For this review, take the finished solid that the model builds, in its own axes (mm). A direction names the side the tool comes from. Coordinates: 2 decimals unless noted, no trailing zeros. Loops run counter-clockwise (first coordinate to the right, second up) from the corner with the lowest first, then second, coordinate; pieces in that order, holes last. Notation, with made-up numbers: (8.25, 48) - (48.25, 48) arc R26 cw to (48.25, 80) - close; hole circle Ø7 at (-30, 49). An arc over 180 degrees is marked (long way). Use one line per item in the form item = value. Start each with the question number.
1. Machinability: for faces 4 (the face through (2.75, 10.74, -2.38)), 5 (the face through (2.5, -11, -2)), which of the approach directions +Z, -Z, +X, -X, +Y, -Y give a long, thin tool a straight path to every point of the face, cutting with its end or side? Answer none if there is none.
2. For pin 1 Ø6 at (y, z) = (-18.5, 0) entering from +X; pin 2 Ø1 at (x, z) = (3.5, -2) entering from -Y; pin 3 Ø4 at (y, z) = (-10, -3.5) entering from -X, all flat-tipped, find the tip position at first contact; note any pin that passes through.
3. To check wall thickness, follow probe 1 along Y at (x, z) = (1.8, 0); probe 2 along Z at (x, y) = (4.45, -1); probe 3 along Z at (x, y) = (2.9, 19.5). State the ranges of each line that lie inside material, in increasing order.
4. Draft analysis for pull direction Z (two halves, no side actions). For faces 1 (the face through (1.268, 12.864, 6.691)), 2 (the face through (2.218, -22.804, -2.994)), 3 (the face through (5, 10, -10)), state which applies: +Z half, -Z half, draft (parallel to the pull), parting line (faces both ways), or undercut.
5. Add section A-A on y = 0. Give the boundary of the cut face in (x, z).
6. Add section C-C on x = 1.7. Give the boundary of the cut face in (y, z), and give its area (3 significant figures).
```python
from build123d import *

# Parameters (mm, degrees)
SKETCH_2_R               = 2.25
CUT_EXTRUDE_1_DEPTH      = 33.908965344
PATTERN_CIRCULAR_1_COUNT = 4
CHAMFER_1_SIZE           = 0.5


with BuildPart() as part:
    # Эскиз1 → Повернуть1 (revolve)
    with BuildSketch(Plane.XY, mode=Mode.PRIVATE) as revolve_1_sk:
        Polygon((0, 23), (0, 14.5), (2.5, 14.5), (2.5, 11), (3, 11), (5, 13), (5, 23), align=None)
    revolve(revolve_1_sk.sketch.rotate(Axis((0, 0, 0), (1, 0, 0)), 90), axis=Axis((0, 0, 0), (1, 0, 0)))

    # Эскиз2 → Вырез-Вытянуть1 (cut, through all)
    with BuildSketch(Plane(origin=(5, 0, 0), x_dir=(0, 0, -1), z_dir=(1, 0, 0))):
        with Locations((0, 18.5)):
            Circle(SKETCH_2_R)
    cut_extrude_1 = extrude(amount=-CUT_EXTRUDE_1_DEPTH, mode=Mode.SUBTRACT)

    # Круговой массив1: Вырез-Вытянуть1 ×4 about axis
    pattern_circular_1_axis = Axis((0, 0, 0), (1, 0, 0))
    for i in range(1, PATTERN_CIRCULAR_1_COUNT):
        add(cut_extrude_1.rotate(pattern_circular_1_axis, i * 360 / PATTERN_CIRCULAR_1_COUNT), mode=Mode.SUBTRACT)

    # Фаска1
    chamfer_1_edges = [part.edges().sort_by_distance(p)[0] for p in [
        (5, 0, -23),
    ]]
    chamfer(chamfer_1_edges, length=CHAMFER_1_SIZE)


solid = part.part
```
Conclusion:
q1.face_4 = +X, -X
q1.face_5 = -X
q2.pin_1 = 5
q2.pin_2 = -22.95
q2.pin_3 = 2.5
q3.probe_1 = -23 to -20.75, -16.25 to -14.5, 14.5 to 16.25, 20.75 to 23
q3.probe_2 = -22.98 to -20.52, -16.48 to -12.41, 12.41 to 16.48, 20.52 to 22.98
q3.probe_3 = -12.2 to -2.02, 2.02 to 12.2
q4.face_1 = undercut
q4.face_2 = parting line
q4.face_3 = draft
q5.outline = (0, -23) - (4.5, -23) - (5, -22.5) - (5, -20.75) - (0, -20.75) - close; (0, -16.25) - (5, -16.25) - (5, -13) - (3, -11) - (2.5, -11) - (2.5, -14.5) - (0, -14.5) - close; (0, 14.5) - (2.5, 14.5) - (2.5, 11) - (3, 11) - (5, 13) - (5, 16.25) - (0, 16.25) - close; (0, 20.75) - (5, 20.75) - (5, 22.5) - (4.5, 23) - (0, 23) - close
q6.outline = circle Ø46 at (0, 0); hole circle Ø4.5 at (-18.5, 0); hole circle Ø29 at (0, 0); hole circle Ø4.5 at (0, -18.5); hole circle Ø4.5 at (0, 18.5); hole circle Ø4.5 at (18.5, 0)
q6.area = 938 mm^2
